CAD build for the part. Positions are in the model's coordinates, mm. A direction names the side the tool comes from. Give positions to 0.01 mm unless a question says otherwise; leave off trailing zeros. Order: outer loops, then holes, each group sorted by start corner. A loop starts at its lowest first (then second) coordinate and runs counter-clockwise, first axis right, second up.
Item 1: Which spindle directions (+Z, -Z, +X, -X, +Y, -Y) get a long thin tool onto all of the face, cutting with end or side? Do faces 5 (the flat face through (-386.158, 1214, 1171)), 6 (the flat face through (395, 1238.729, 47)), 7 (the flat face through (490.142, 1252, 1171)), 8 (the flat face through (337.286, 1237, 1171)), 9 (the flat face through (39, 1284.029, 856)). Say none if no direction does.
Item 2: Wall check: L1, parallel to Z at x = 430, y = 1258; L2, parallel to X at y = 1269, z = 243; L3, parallel to X at y = 1261, z = 684. Give the ranges that are in metal, low to high.
Item 3: Band-saw the part on C-C on x = 395.5. Give the cut face in (y, z), plus the area to 3 significant figures.
Item 4: Band-saw the part on B-B on y = 1352.5. Give the cut face in (x, z), plus the area to 3 significant figures.
Item 5: Flat gauge pins, fed straight in: P1, Ø12, axis at x = -76, y = 1298.5, coming from the -Z side; P2, Ø14, axis at x = -392.5, z = 598, coming from the -Y side; P3, Ø3, axis at y = 1289.5, z = 911.5, coming from the +X side; P4, Ø22.5, axis at y = 1246, z = 66.5, coming from the -X side. Where does each tip first touch, or does it go through?
Item 6: Band-saw the part on A-A on z = 775. Give the cut face in (x, y).
Item 7: Two-plate mould, pull along Z, no slides. Class faces 1 (the flat face through (39, 1206, 95.714)), 2 (the flat face through (-398.858, 1251, 1171)), 3 (the flat face through (43, 1209, 0)), 4 (the flat face through (546, 1284.029, 607)): released by +Z, released by -Z, zero draft, split by the parting line, or undercut.
Item 8: Band-saw the part on D-D on x = 27.5. Give the cut face in (y, z), plus the area to 3 significant figures.
```python
from build123d import *

# Parameters (mm, degrees)
EXTRUDE1_DEPTH = 1219.2
SKETCH2_W      = 943.681413061
SKETCH2_H      = 390.553297683
EXTRUDE2_DEPTH = 1365.086621936
EXTRUDE3_REACH = 2095.85


with BuildPart() as part:
    # Sketch1 → Extrude1 (new body)
    with BuildSketch(Plane(origin=(0, 0, 0), x_dir=(-1, 0, 0), z_dir=(0, 0, 1))):
        Polygon((-604.441999719, -1264.128861053), (-490.141999719, -1264.128861053), (-490.141999719, -1238.728861053), (-477.441999719, -1238.728861053), (-477.441999719, -1189.511943694), (-409.740815056, -1189.511943694), (-409.740815056, -1214.120402374), (-432.600815056, -1214.120402374), (-432.600815056, -1238.728861053), (-356.400815056, -1238.728861053), (-356.400815056, -1214.120402374), (-379.260815056, -1214.120402374), (-379.260815056, -1189.511943694), (287.976815619, -1189.511943694), (287.976815619, -1214.120402374), (265.116815619, -1214.120402374), (265.116815619, -1238.728861053), (341.316815619, -1238.728861053), (341.316815619, -1214.120402374), (318.456815619, -1214.120402374), (318.456815619, -1189.511943694), (386.158000281, -1189.511943694), (386.158000281, -1238.728861053), (398.858000281, -1238.728861053), (398.858000281, -1264.128861053), (513.158000281, -1264.128861053), (513.158000281, -1284.029355434), (365.129820759, -1284.029355434), (365.129820759, -1259.541912826), (246.001721585, -1259.541912826), (246.001721585, -1214.120402374), (-337.285721023, -1214.120402374), (-337.285721023, -1259.541912826), (-456.413820196, -1259.541912826), (-456.413820196, -1284.029355434), (-604.441999719, -1284.029355434), align=None)
    extrude(amount=EXTRUDE1_DEPTH)

    # Sketch2 → Extrude2 (cut, through all)
    with BuildSketch(Plane(origin=(0, 1284.029355434, 0), x_dir=(1, 0, 0), z_dir=(0, 1, 0))):
        with Locations((45.641999718, -290.990730837)):
            Rectangle(SKETCH2_W, SKETCH2_H)
        with Locations((45.641999718, -928.209269163)):
            Rectangle(SKETCH2_W, SKETCH2_H)
    extrude(amount=-EXTRUDE2_DEPTH, mode=Mode.SUBTRACT)

    # Extrude3: up to this face of the body (flat: up to its plane)
    extrude3_end = Plane(part.part.faces().sort_by_distance((604.441999719, 1274.079108244, 609.6))[0])
    # Sketch3 → Extrude3 (add, up to the picked face)
    with BuildSketch(Plane.ZY.offset(513.158000281), mode=Mode.PRIVATE) as extrude3_sk1:
        Polygon((309.974780867, 1284.029355434), (309.974780867, 1333.517105863), (269.543425995, 1333.517105863), (269.543425995, 1392.72016121), (415.385098923, 1392.72016121), (415.385098923, 1284.029355434), align=None)
    extrude3_tool1 = split(extrude(extrude3_sk1.sketch, amount=-EXTRUDE3_REACH, mode=Mode.PRIVATE), bisect_by=extrude3_end, keep=Keep.BOTH, mode=Mode.PRIVATE)
    # Sketch3 → Extrude3 (add, up to the picked face)
    with BuildSketch(Plane.ZY.offset(513.158000281), mode=Mode.PRIVATE) as extrude3_sk2:
        Polygon((803.814901077, 1284.029355434), (909.225219133, 1284.029355434), (909.225219133, 1333.517105863), (949.656574005, 1333.517105863), (949.656574005, 1392.72016121), (803.814901077, 1392.72016121), align=None)
    extrude3_tool2 = split(extrude(extrude3_sk2.sketch, amount=-EXTRUDE3_REACH, mode=Mode.PRIVATE), bisect_by=extrude3_end, keep=Keep.BOTH, mode=Mode.PRIVATE)
    add(extrude3_tool1.solids().sort_by(Axis((-513.158, 1342.650934, 350.077941), (1, 0, 0)))[0])
    add(extrude3_tool2.solids().sort_by(Axis((-513.158, 1342.650934, 869.122059), (1, 0, 0)))[0])


solid = part.part
```
The answers:
1. face 5: +Z, -Z, -X, -Y
1. face 6: +Z, -Z
1. face 7: +Z, -Z, +X, -Y
1. face 8: +Z, -Z, +Y
1. face 9: -Y
2. L1: z = 0 to 95.71, 486.27 to 732.93, 1123.49 to 1219.2
2. L2: x = -513.16 to -426.2, 517.48 to 604.44
2. L3: x = -398.86 to -365.13, 456.41 to 490.14
3. outline: (1238.73, 0) - (1259.54, 0) - (1259.54, 95.71) - (1238.73, 95.71) - close; (1238.73, 486.27) - (1259.54, 486.27) - (1259.54, 732.93) - (1238.73, 732.93) - close; (1238.73, 1123.49) - (1259.54, 1123.49) - (1259.54, 1219.2) - (1238.73, 1219.2) - close; (1284.03, 309.97) - (1333.52, 309.97) - (1333.52, 269.54) - (1392.72, 269.54) - (1392.72, 415.39) - (1284.03, 415.39) - close; (1284.03, 803.81) - (1392.72, 803.81) - (1392.72, 949.66) - (1333.52, 949.66) - (1333.52, 909.23) - (1284.03, 909.23) - close
3. area: 36,800 mm2
4. outline: (-513.16, 269.54) - (604.44, 269.54) - (604.44, 415.39) - (-513.16, 415.39) - close; (-513.16, 803.81) - (604.44, 803.81) - (604.44, 949.66) - (-513.16, 949.66) - close
4. area: 326,000 mm2
5. P1: stops at z = 309.97
5. P2: stops at y = 1189.51
5. P3: passes through
5. P4: stops at x = -398.86
6. outline: (-513.16, 1264.13) - (-426.2, 1264.13) - (-426.2, 1284.03) - (-513.16, 1284.03) - close; (517.48, 1264.13) - (604.44, 1264.13) - (604.44, 1284.03) - (517.48, 1284.03) - close
7. face 1: undercut
7. face 2: zero draft
7. face 3: released by -Z
7. face 4: undercut
8. outline: (1189.51, 0) - (1214.12, 0) - (1214.12, 95.71) - (1189.51, 95.71) - close; (1189.51, 486.27) - (1214.12, 486.27) - (1214.12, 732.93) - (1189.51, 732.93) - close; (1189.51, 1123.49) - (1214.12, 1123.49) - (1214.12, 1219.2) - (1189.51, 1219.2) - close; (1284.03, 309.97) - (1333.52, 309.97) - (1333.52, 269.54) - (1392.72, 269.54) - (1392.72, 415.39) - (1284.03, 415.39) - close; (1284.03, 803.81) - (1392.72, 803.81) - (1392.72, 949.66) - (1333.52, 949.66) - (1333.52, 909.23) - (1284.03, 909.23) - close
8. area: 38,500 mm2
